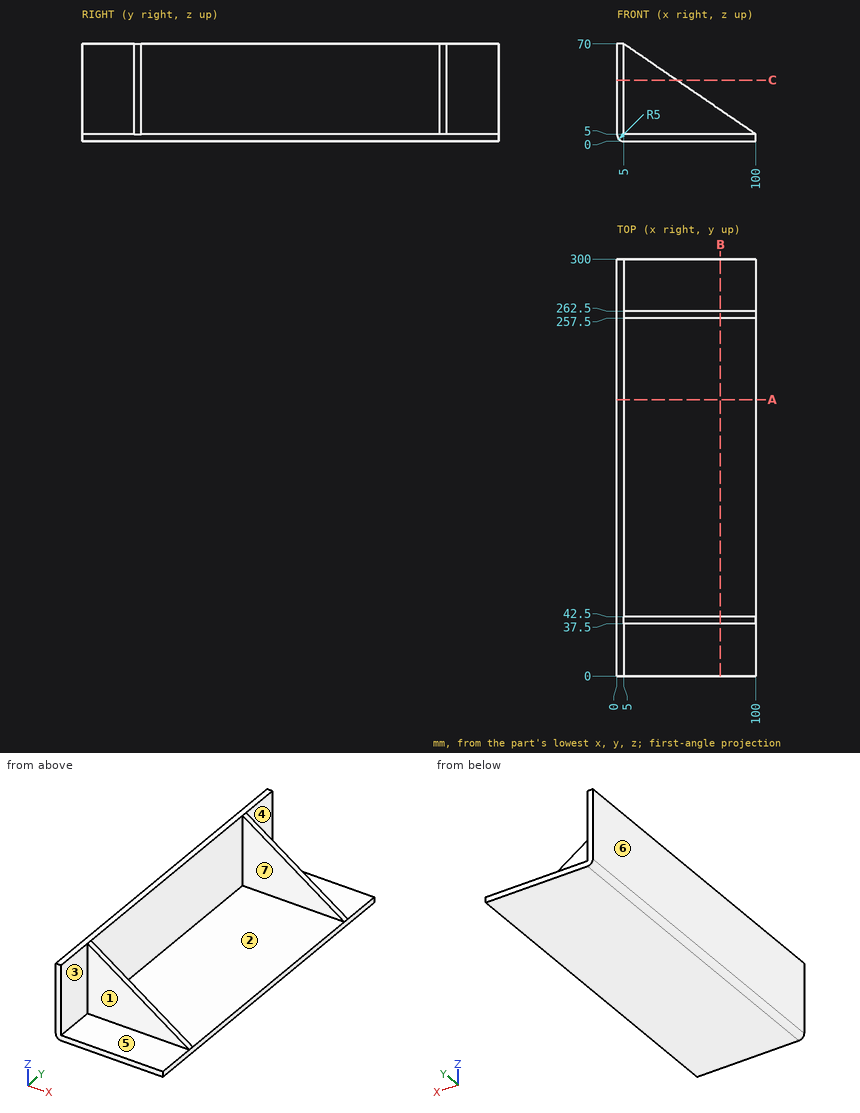
The figure shows three views and two pictorial views of one solid part (mm, origin at its lowest corner). Answer the questions. A direction names the side the tool comes from. Give positions to 0.01 mm unless a question says otherwise; leave off trailing zeros. Order: outer loops, then holes, each group sorted by start corner. A loop starts at its lowest first (then second) coordinate and runs counter-clockwise, first axis right, second up. Notation, with made-up numbers: (-22, -35.5) -> (23, -35.5) arc R22 cw to (23, -4.5) -> close; hole circle Ø7 at (66, -15). An arc over 180 degrees is marked (long way). Write each question's results on one line, items separated by ' | '.
Q1. The part is cut by section B-B, the plane x = 74.5. Give the vertices of the cut face in (y, z), and give its area (3 significant figures).
Checked values:
outline: (0, 0) -> (300, 0) -> (300, 5) -> (262.5, 5) -> (262.5, 22.45) -> (257.5, 22.45) -> (257.5, 5) -> (42.5, 5) -> (42.5, 22.45) -> (37.5, 22.45) -> (37.5, 5) -> (0, 5) -> close | area: 1,670 mm^2
Q2. Determine the mould class of the marked faces 1, 2 and 3 for opening direction Y: pulls with the +Y half, pulls with the -Y half, needs draft (parallel to the pull), parting line crosses it, or undercut.
Checked values:
face 1: pulls with the -Y half | face 2: undercut | face 3: needs draft
Q3. The part is cut by section C-C, the plane z = 44. Give the vertices of the cut face in (x, y), and give its area (3 significant figures).
Checked values:
outline: (0, 0) -> (5, 0) -> (5, 37.5) -> (43, 37.5) -> (43, 42.5) -> (5, 42.5) -> (5, 257.5) -> (43, 257.5) -> (43, 262.5) -> (5, 262.5) -> (5, 300) -> (0, 300) -> close | area: 1,880 mm^2
Q4. The part is cut by section A-A, the plane y = 199. Give the vertices of the cut face in (x, z).
Checked values:
outline: (0, 5) arc R5 ccw to (5, 0) -> (100, 0) -> (100, 5) -> (5, 5) -> (5, 70) -> (0, 70) -> close
Q5. Straight lines are drawn through the part: probe 1 along Y at (x, z) = (62.5, 7); probe 2 along X at (y, z) = (239.5, 24.5). For each, find the intervals that lie inside material, in ascending order. Write a range as from..to.
Checked values:
probe 1: y = 37.5..42.5, 257.5..262.5 | probe 2: x = 0..5
Q6. Which of the six approach directions +Z, -Z, +X, -X, +Y, -Y give full straight-line access (tool end or side, diameter ignored) to the marked faces 4, 5, 6 and 7?
Checked values:
face 4: +Z, +X, +Y | face 5: +Z, +X, -Y | face 6: +Z, -Z, -X, +Y, -Y | face 7: +Z, +X
Q7. Each of these flat-tipped pins is pushed along its axis until it touches: P1, Ø1, axis at y = 57.5, z = 25, coming from the +X side; P2, Ø6, axis at x = 68, y = 36.5, coming from the +Z side; P3, Ø19.5, axis at x = 54, z = 27.5, coming from the +Y side. Where does it stop, or does it pass through?
Checked values:
P1: stops at x = 5 | P2: stops at z = 28.83 | P3: stops at y = 262.5
